from build123d import *

# Parameters (mm, degrees)
SKETCH1_W                     = 80
SKETCH1_H                     = 80
PCB_DEPTH                     = 2
SKETCH3_W                     = 62
SKETCH3_H                     = 34
BATTERY_STACK_DEPTH           = 10
LPATTERN3_COUNT               = 2
LPATTERN3_PITCH               = 41
SKETCH4_R                     = 1.8
ATTACHMENT_HOLES_DEPTH        = 3
SKETCH6_R                     = 1.5875
BATTERY_CABLE_TIE_HOLES_DEPTH = 3
LPATTERN2_COUNT               = 2
LPATTERN2_PITCH               = 35
LPATTERN2_COUNT_DIR2          = 3
LPATTERN2_PITCH_DIR2          = 40


with BuildPart() as part:
    # Sketch1 → PCB (new body)
    with BuildSketch(Plane(origin=(0, 0, 0), x_dir=(1, 0, 0), z_dir=(0, 1, 0))):
        with Locations((40, 40)):
            Rectangle(SKETCH1_W, SKETCH1_H)
    extrude(amount=PCB_DEPTH)

    # Sketch3 → Battery Stack (add)
    with BuildSketch(Plane(origin=(0, 2, 0), x_dir=(1, 0, 0), z_dir=(0, 1, 0))):
        with Locations((39, 19)):
            Rectangle(SKETCH3_W, SKETCH3_H)
    battery_stack = extrude(amount=BATTERY_STACK_DEPTH)

    # LPattern3: Battery Stack ×2
    with Locations(*[(0, 0, -i * LPATTERN3_PITCH) for i in range(1, LPATTERN3_COUNT)]):
        add(battery_stack)

    # Sketch4 → Attachment holes (cut, through all)
    with BuildSketch(Plane(origin=(0, 2, 0), x_dir=(1, 0, 0), z_dir=(0, 1, 0))):
        with Locations((5, 75)):
            Circle(SKETCH4_R)
        with Locations((75, 75)):
            Circle(SKETCH4_R)
        with Locations((75, 5)):
            Circle(SKETCH4_R)
        with Locations((5, 5)):
            Circle(SKETCH4_R)
    extrude(amount=-ATTACHMENT_HOLES_DEPTH, mode=Mode.SUBTRACT)

    # Sketch6 → Battery Cable Tie Holes (cut, through all)
    with BuildSketch(Plane(origin=(0, 2, 0), x_dir=(1, 0, 0), z_dir=(0, 1, 0))):
        with Locations((20, 0)):
            Circle(SKETCH6_R)
    battery_cable_tie_holes = extrude(amount=-BATTERY_CABLE_TIE_HOLES_DEPTH, mode=Mode.SUBTRACT)

    # LPattern2: Battery Cable Tie Holes 2 × 3
    with Locations(*[(i * LPATTERN2_PITCH, 0, -j * LPATTERN2_PITCH_DIR2) for i in range(LPATTERN2_COUNT) for j in range(LPATTERN2_COUNT_DIR2) if (i, j) != (0, 0)]):
        add(battery_cable_tie_holes, mode=Mode.SUBTRACT)


solid = part.part
Input: part model. Units: mm. Frame: model coordinates. A direction names the side the tool comes from. Coordinates: 2 decimals unless noted, no trailing zeros. Order: outer loops, then holes, each group sorted by start corner. A loop starts at its lowest first (then second) coordinate and runs counter-clockwise, first axis right, second up.
1. Draft query along Z for faces 4 (the cylindrical face through (54.965, 1.014, -78.413)), 5 (the flat face through (70, 7, -60)), 6 (the cylindrical face through (55.035, 1.014, -1.587)), 7 (the flat face through (39, 7, -43)). Return one class per face: +Z half, -Z half, draft (parallel to the pull), parting line (faces both ways), or undercut.
Checked values:
face 4: -Z half
face 5: draft
face 6: +Z half
face 7: undercut
2. Cut plane C-C, the plane z = -75. Return loops of the section in (x, y).
Checked values:
outline: (0, 0) - (3.2, 0) - (3.2, 2) - (0, 2) - close; (6.8, 0) - (73.2, 0) - (73.2, 2) - (70, 2) - (70, 12) - (8, 12) - (8, 2) - (6.8, 2) - close; (76.8, 0) - (80, 0) - (80, 2) - (76.8, 2) - close
3. Contact query for flat-ended pins moving along their axis: P1, Ø5, axis at x = 47, y = 8, coming from the +Z side; P2, Ø4, axis at y = 7.5, z = -49.5, coming from the -X side; P3, Ø3.5, axis at x = 20, z = -40, coming from the +Y side. Output: stop coordinate, or through.
Checked values:
P1: stops at z = -2
P2: stops at x = 8
P3: stops at y = 2
4. Cut plane A-A, the plane y = 10.5. Return loops of the section in (x, z).
Checked values:
outline: (8, -77) - (70, -77) - (70, -43) - (8, -43) - close; (8, -36) - (70, -36) - (70, -2) - (8, -2) - close
5. Ray query, line 1 along X through (y, z) = (1.05, -75); line 2 along Z through (x, y) = (75, 1.6); line 3 along Z through (x, y) = (20, 0.95). Return the intervals inside material, ascending.
Checked values:
line 1: x = 0 to 3.2, 6.8 to 73.2, 76.8 to 80
line 2: z = -80 to -76.8, -73.2 to -6.8, -3.2 to 0
line 3: z = -78.41 to -41.59, -38.41 to -1.59
6. Cut plane D-D, the plane x = 5. Return loops of the section in (y, z), plus the area to 3 significant figures.
Checked values:
outline: (0, -80) - (2, -80) - (2, -76.8) - (0, -76.8) - close; (0, -73.2) - (2, -73.2) - (2, -6.8) - (0, -6.8) - close; (0, -3.2) - (2, -3.2) - (2, 0) - (0, 0) - close
area: 146 mm2
7. Cut plane B-B, the plane x = 55. Return loops of the section in (y, z), plus the area to 3 significant figures.
Checked values:
outline: (0, -78.41) - (2, -78.41) - (2, -77) - (12, -77) - (12, -43) - (2, -43) - (2, -41.59) - (0, -41.59) - close; (0, -38.41) - (2, -38.41) - (2, -36) - (12, -36) - (12, -2) - (2, -2) - (2, -1.59) - (0, -1.59) - close
area: 827 mm2
8. Access query for faces 1 (the flat face through (8, 7, -19)), 2 (the flat face through (39, 7, -77)), 3 (the flat face through (39, 7, -36)). Directions: +Z, -Z, +X, -X, +Y, -Y. A direction counts if a zero-diameter tool reaches every point of the face in a straight line with its end or side. Return the directions, or none.
Checked values:
face 1: +Z, -Z, -X, +Y
face 2: -Z, +X, -X, +Y
face 3: +X, -X, +Y
